Autodesk Inventor part; units mm, degrees
ref_plane "YZ Plane" through (0, 0, 0) normal (1, 0, 0) x (0, 1, 0)
ref_plane "XZ Plane" through (0, 0, 0) normal (0, 1, 0) x (-1, 0, 0)
ref_plane "XY Plane" through (0, 0, 0) normal (0, 0, 1) x (1, 0, 0)
sketch "Sketch1" plane through (0, 0, 0) normal (0, 1, 0) x (-1, 0, 0)
  line L0 (-50.8, 26.67) -> (-50.8, -26.67)
  line L1 (-50.8, -26.67) -> (50.8, -26.67)
  line L2 (50.8, -26.67) -> (50.8, 26.67)
  line L3 (50.8, 26.67) -> (-50.8, -26.67) construction
  line L4 (50.8, -26.67) -> (-50.8, 26.67) construction
  line L5 (51.8, 28.17) -> (-51.8, 28.17)
  line L6 (-51.8, 28.17) -> (-51.8, -28.17)
  line L7 (-51.8, -28.17) -> (51.8, -28.17)
  line L8 (51.8, -28.17) -> (51.8, 28.17)
  line L9 (51.8, 28.17) -> (-51.8, -28.17) construction
  line L10 (-51.8, 28.17) -> (51.8, -28.17) construction
  line L11 (-54.8, 31.17) -> (54.8, 31.17)
  line L12 (54.8, 31.17) -> (54.8, -31.17)
  line L13 (54.8, -31.17) -> (-54.8, -31.17)
  line L14 (-54.8, -31.17) -> (-54.8, 31.17)
  line L15 (-54.8, 31.17) -> (54.8, -31.17) construction
  line L16 (54.8, 31.17) -> (-54.8, -31.17) construction
  line L17 (54.8, -31.17) -> (-5.2, -31.17)
  line L18 (-5.2, -31.17) -> (-5.2, -51.17)
  line L19 (-5.2, -51.17) -> (54.8, -51.17)
  line L20 (54.8, -51.17) -> (54.8, -31.17)
  line L21 (54.8, -51.17) -> (34.8, -51.17)
  line L22 (-41.91, -26.67) -> (-36.83, -26.67)
  line L23 (38.1, -26.67) -> (33.02, -26.67)
  line L24 (54.8, -51.17) -> (34.8, -51.17)
  line L25 (34.8, -51.17) -> (34.8, 53.17)
  line L26 (34.8, 53.17) -> (54.8, 53.17)
  line L27 (54.8, 53.17) -> (54.8, -51.17)
  line L28 (-50.8, 26.67) -> (50.8, 26.67)
  point P0 (0, 0)
  point P1 (36.83, 24.13)
  point P2 (-45.72, 24.13)
  point P3 (-45.72, 24.13)
  point P4 (-39.37, -24.13)
  point P5 (35.56, -24.13)
  point P6 (0, 0)
  point P7 (0, 0)
  dimension "d0" = 101.6
  dimension "d1" = 53.34
  dimension "d2" = 13.97
  dimension "d4" = 96.52
  dimension "d5" = 90.17
  dimension "d7" = 15.24
  dimension "d8" = 101.6
  dimension "d11" = 103.6
  dimension "d12" = 56.34
  dimension "d13" = 62.34
  dimension "d14" = 109.6
  dimension "d15" = 20
  dimension "d25" = 60
  dimension "d31" = 20
  dimension "d33" = 0
  dimension "d60" = 25
extrude "Extrusion1" add sketch "Sketch1" against normal blind 3
extrude "Extrusion2" add sketch "Sketch1" along normal blind 5 contours L25 L11 L12 L13 L7 L8 L5 | L5 L6 L7 L25 L13 L14 L11
extrude "Extrusion6" add sketch "Sketch1" along normal blind 3 contours L0 L1 L25 L7 L6 L5 L28 | L25 L5 L8 L7 L1 L2 L28
sketch "Sketch5" plane through (0, 0, 0) normal (0, 1, 0) x (1, 0, 0)
  line L0 (50.8, -26.67) -> (-50.8, -26.67)
  arc A0 (-33.33, -24.13) -> (-40.33, -24.13) centre (-36.83, -24.13) ccw
  line L1 (-33.33, -24.13) -> (-33.33, -26.67)
  line L2 (-33.33, -26.67) -> (-40.33, -26.67)
  line L3 (-40.33, -26.67) -> (-40.33, -24.13)
  arc A1 (49.22, -24.13) -> (42.22, -24.13) centre (45.72, -24.13) ccw
  line L4 (42.22, -24.13) -> (42.22, -26.67)
  line L5 (-50.8, -26.67) -> (50.8, -26.67)
  line L6 (49.22, -24.13) -> (49.22, -26.67)
  line L7 (49.22, -26.67) -> (42.22, -26.67)
  arc A2 (35.87, 24.13) -> (42.87, 24.13) centre (39.37, 24.13) ccw
  line L8 (35.87, 24.13) -> (35.87, 26.67)
  line L9 (50.8, 26.67) -> (-50.8, 26.67)
  line L10 (35.87, 26.67) -> (42.87, 26.67)
  line L11 (42.87, 26.67) -> (42.87, 24.13)
  arc A3 (-39.06, 24.13) -> (-32.06, 24.13) centre (-35.56, 24.13) ccw
  line L12 (-39.06, 24.13) -> (-39.06, 26.67)
  line L13 (-39.06, 26.67) -> (-32.06, 26.67)
  line L14 (-32.06, 26.67) -> (-32.06, 24.13)
  point P0 (0, 0)
  dimension "d64" = 7
  dimension "d65" = 7
  dimension "d68" = 7
  dimension "d69" = 7
  dimension "d70" = 7
extrude "Extrusion7" add sketch "Sketch5" along normal blind 1
hole "Hole3" at (-36.83, 0, 24.13) at (-35.56, 0, -24.13) at (39.37, 0, -24.13) at (45.72, 0, 24.13) direction (0, -1, 0) diameter 3.8 end through all
sketch "Sketch6" plane through (0, 1, 0) normal (0, 1, 0) x (1, 0, 0)
  point P0 (0, 0)
  point P1 (-36.83, -24.13)
  point P2 (-35.56, 24.13)
  point P3 (39.37, 24.13)
  point P4 (45.72, -24.13)
hole "Hole4" at (-36.83, 1, 24.13) at (-35.56, 1, -24.13) at (39.37, 1, -24.13) at (45.72, 1, 24.13) direction (0, -1, 0) diameter 3.8 end through all
fillet "Fillet1" radius 25 1 edges at (-34.8, -1.5, 31.17)
fillet "Fillet2" radius 20 1 edges at (5.2, -1.5, -31.17)
fillet "Fillet3" radius 5 2 edges at (5.2, -1.5, -51.17) (-9.9807, -1.5, 31.17)
sketch "Sketch2" plane through (0, 0, 0) normal (0, 1, 0) x (1, 0, 0)
  line L0 (-34.8, -53.17) -> (-54.8, -53.17)
  line L1 (5.2, 31.17) -> (5.2, 51.17)
  line L2 (-54.8, 51.17) -> (-34.8, 51.17)
  circle A0 centre (-44.8, -48.17) radius 5
  circle A1 centre (-44.8, 41.17) radius 5
  circle A2 centre (-4.8, 41.17) radius 5
  line L3 (-49.8, -48.17) -> (-49.8, -53.17)
  line L4 (-39.8, -48.17) -> (-39.8, -53.17)
  line L5 (-34.8, -53.17) -> (-54.8, -53.17)
  line L6 (-39.8, -53.17) -> (-49.8, -53.17)
  line L7 (-54.8, 31.17) -> (-54.8, 51.17)
  line L8 (-54.8, -53.17) -> (-54.8, -31.17)
  point P0 (0, 0)
  point P1 (-36.8, -56.83)
  dimension "d35" = 5
  dimension "d37" = 10
  dimension "d38" = 10
  dimension "d39" = 10
  dimension "d40" = 10
  dimension "d41" = 10
  dimension "d42" = 10
  dimension "d85" = 10
  dimension "d86" = 10
hole "Hole5" at (-44.8, 0, 48.17) at (-4.8, 0, -41.17) direction (0, -1, 0) diameter 3.5 end through all
sketch "Sketch3" plane through (-44.8, 2, 48.17) normal (0, 1, 0) x (-1, 0, 0)
  arc A0 (-5, 0) -> (5, 0) centre (0, 0) ccw
  circle A1 centre (0, -89.34) radius 5
  circle A2 centre (-40, -89.34) radius 5
  line L0 (5, 5) -> (-5, 5)
  line L1 (-5, 5) -> (-5, 0)
  line L2 (5, 0) -> (5, 5)
  point P0 (-44.8, -48.17)
properties part number "support arduino_v2"
CAD build for the part. Positions are in the model's coordinates, mm. A direction names the side the tool comes from. Round coordinates to 2 decimals unless told otherwise and drop trailing zeros. Write each loop counter-clockwise with the first axis right and the second up, starting at its lowest first coordinate (ties: lowest second). Pieces come first, ordered by that corner, then holes. Notation, with made-up numbers: M 77.5,-32.5 L 114.5,-32.5 A16 cw 114.5,-5.5 Z; hole C 28,-7.5 d9. An arc over 180 degrees is marked long. Use a Markdown table: item, result. Add a question column.
1. Flat gauge pins, fed straight in: P1, Ø11, axis at x = -24, z = 37.5, coming from the +Y side; P2, Ø4, axis at x = -15, y = 4, coming from the +Z side; P3, Ø1.6, axis at x = 19, y = 4, coming from the -Z side. Where does each tip first touch, or does it go through?
2. Drill centre lines: probe 1 along X at (y, z) = (-0.55, 24.13); probe 2 along Z at (x, y) = (13.5, 4.5); probe 3 along X at (y, z) = (-0.85, -24.13). Where is each one in solid material? Low to high.
3. Slice it at B-B on z = -41.17. Give the cut face in (x, y), then the cut area to 3 significant figures.
4. Slice it at C-C on z = 3.5. Give the cut face in (x, y).
5. Slice it at D-D on x = 34. Give the cut face in (y, z), then the cut area to 3 significant figures.
6. Slice it at A-A on x = 45.72. Give the cut face in (y, z), then the cut area to 3 significant figures.
7. 3-axis set-ups, long thin cutter, end or side, ignore diameter. For faces 1 (the face through (-4.13, -1.521, -39.553)), 2 (the face through (-36.91, 0.49, 20.63)), 3 (the face through (1, 2, 31.17)): which of +Z, -Z, +X, -X, +Y, -Y reach the whole face in a straight line?
8. Pull direction X, two halves, no side cores. Call faces 4 (the face through (-11, -3, 2)), 5 (the face through (-35.48, 0.49, -20.63)), 6 (the face through (54.8, 1, 0)): released by +X, released by -X, zero draft, split by the parting line, or undercut.
Reply:
| question | item | result |
|---|---|---|
| 1 | P1 | stops at y = 0 |
| 1 | P2 | stops at z = 31.17 |
| 1 | P3 | stops at z = -31.17 |
| 2 | probe 1 | x = -54.8 to -38.73, -34.93 to 43.82, 47.62 to 54.8 |
| 2 | probe 2 | z = -31.17 to -28.17, 28.17 to 31.17 |
| 2 | probe 3 | x = -54.8 to -37.46, -33.66 to 37.47, 41.27 to 54.8 |
| 3 | outline | M -54.8,-3 L -6.55,-3 L -6.55,0 L -54.8,0 Z; M -3.05,-3 L 7.88,-3 L 7.88,0 L -3.05,0 Z |
| 3 | area | 178 mm^2 |
| 4 | outline | M -54.8,-3 L 54.8,-3 L 54.8,5 L 51.8,5 L 51.8,3 L 50.8,3 L 50.8,0 L -50.8,0 L -50.8,3 L -51.8,3 L -51.8,5 L -54.8,5 Z |
| 5 | outline | M -3,-31.17 L 5,-31.17 L 5,-28.17 L 3,-28.17 L 3,-26.67 L 0,-26.67 L 0,26.67 L 3,26.67 L 3,28.17 L 5,28.17 L 5,31.17 L -3,31.17 Z |
| 5 | area | 226 mm^2 |
| 6 | outline | M -3,-31.17 L 5,-31.17 L 5,-28.17 L 3,-28.17 L 3,-26.67 L 0,-26.67 L 0,20.63 L 1,20.63 L 1,22.23 L -3,22.23 Z; M -3,26.03 L 1,26.03 L 1,26.67 L 3,26.67 L 3,28.17 L 5,28.17 L 5,31.17 L -3,31.17 Z |
| 6 | area | 217 mm^2 |
| 7 | face 1 | +Y, -Y |
| 7 | face 2 | +Y |
| 7 | face 3 | +Z, +X, +Y |
| 8 | face 4 | zero draft |
| 8 | face 5 | undercut |
| 8 | face 6 | released by +X |
